Could you check a few things on this model? Use its own coordinates, in mm. A direction names the side the tool comes from. Give positions to 0.01 mm unless a question says otherwise; leave off trailing zeros. Loops run counter-clockwise (first coordinate to the right, second up) from the corner with the lowest first, then second, coordinate; pieces in that order, holes last.
1. For faces 5 (the flat face through (0, 0, 0)), 6 (the flat face through (0, -59, -31.241)), 7 (the cylindrical face through (-24.32, -60.25, -30.49)), which set-ups out of +Z, -Z, +X, -X, +Y, -Y let a thin tool reach every point of the face, with its end or its side?
2. Imagine slicing it at A-A (x = 20). List the corners of the cut face in (y, z) for me.
3. Thinking about a two-plate mould opening in Z: for faces 1 (the cylindrical face through (-26.109, -60.282, 32.238)), 2 (the cylindrical face through (-26.109, -60.282, -32.238)), 3 (the cylindrical face through (24.28, -60.25, -30.53)), 4 (the flat face through (22.535, -59, 32)), which applies, +Z half, -Z half, draft (parallel to the pull), parting line (faces both ways), or undercut?
4. I need wall thicknesses on line 1 along X through (y, z) = (-30.5, -9); line 2 along Y through (x, z) = (-20.5, -11.5); line 3 along Z through (x, y) = (13.5, -26.5). Which ranges of each line are inside material? Lowest first, please.
5. Imagine slicing it at B-B (z = -14.5). List the corners of the cut face in (x, y) for me.
6. Imagine slicing it at C-C (y = -95). List the corners of the cut face in (x, z) for me, plus the area to 3 significant figures.
7. For P1, Ø13.5, axis at x = 10.5, y = -39.5, coming from the +Z side; P2, Ø2, axis at x = 18.5, z = 7, coming from the +Y side; P3, Ø0.8, axis at y = -49.5, z = 32.5, coming from the +X side; P4, Ø0.8, axis at y = -70, z = 33, coming from the -X side, each with a flat end and sliding along its axis, tell me the tip position at first contact or that it passes through.
```python
from build123d import *

# Parameters (mm, degrees)
F0_W     = 55.0703965127
F0_H     = 67.4825981259
F1_DEPTH = 118.9
F2_R     = 5
F3_T     = -2.5


# Not quite as in the source:
# - a shell that OpenCascade refuses in one call is made with other operations: the cavity is built on its own and cut out


with BuildPart() as f1:
    # F0 (on Front) → F1 (new body)
    with BuildSketch(Plane.XZ):
        Rectangle(F0_W, F0_H)
    extrude(amount=F1_DEPTH)

    # F2
    f2_edges = [f1.edges().sort_by_distance(p)[0] for p in [
        (-27.535198, -59.45, 33.741299),
        (27.535198, -59.45, 33.741299),
        (-27.535198, -59.45, -33.741299),
        (27.535198, -59.45, -33.741299),
    ]]
    fillet(f2_edges, radius=F2_R)

    # F3: a shell. OpenCascade refuses it in one call, so the cavity is built on its own and cut out:
    # the body offset inwards by the wall thickness, plus a prism from it out through each open face.
    f3_core = offset(f1.part, amount=F3_T, mode=Mode.PRIVATE)
    f3_exits = [f3_core.faces().sort_by_distance(p)[0] for p in [
        (0, -59.45, 31.241299),
    ]]
    add(f3_core, mode=Mode.SUBTRACT)
    extrude(f3_exits, amount=-F3_T, mode=Mode.SUBTRACT)


solid = f1.part
```
Derived:
1. face 5: +Z, -Z, +X, -X, +Y
1. face 6: +Z
1. face 7: none
2. outline: (-118.9, -33.74) - (0, -33.74) - (0, 33.74) - (-2.5, 33.74) - (-2.5, -31.24) - (-116.4, -31.24) - (-116.4, 33.74) - (-118.9, 33.74) - close
3. face 1: +Z half
3. face 2: -Z half
3. face 3: undercut
3. face 4: draft
4. line 1: x = -27.54 to -25.04, 25.04 to 27.54
4. line 2: y = -118.9 to -116.4, -2.5 to 0
4. line 3: z = -33.74 to -31.24
5. outline: (-27.54, -118.9) - (27.54, -118.9) - (27.54, 0) - (-27.54, 0) - close; hole (-25.04, -116.4) - (25.04, -116.4) - (25.04, -2.5) - (-25.04, -2.5) - close
6. outline: (-27.54, -28.74) arc R5 ccw to (-22.54, -33.74) - (22.54, -33.74) arc R5 ccw to (27.54, -28.74) - (27.54, 28.74) arc R5 ccw to (22.54, 33.74) - (22.54, 31.24) arc R2.5 cw to (25.04, 28.74) - (25.04, -28.74) arc R2.5 cw to (22.54, -31.24) - (-22.54, -31.24) arc R2.5 cw to (-25.04, -28.74) - (-25.04, 28.74) arc R2.5 cw to (-22.54, 31.24) - (-22.54, 33.74) arc R5 ccw to (-27.54, 28.74) - close
6. area: 459 mm2
7. P1: stops at z = -31.24
7. P2: stops at y = 0
7. P3: stops at x = 26.24
7. P4: stops at x = -25.71
